Print and shaded views of the part. All mm, measured from the part's lowest x, y and z. Give positions to 0.01 mm unless a question says otherwise; leave off trailing zeros. Loops run counter-clockwise (first coordinate to the right, second up) from the corner with the lowest first, then second, coordinate; pieces in that order, holes last. Notation, with made-up numbers: M -0.75,72.5 L 34.25,72.5 A23 ccw 34.25,111.5 Z; hole C 55.25,89 d10. An arc over 180 degrees is marked long. Put each result on its own line as item: value. Start each with the question number.
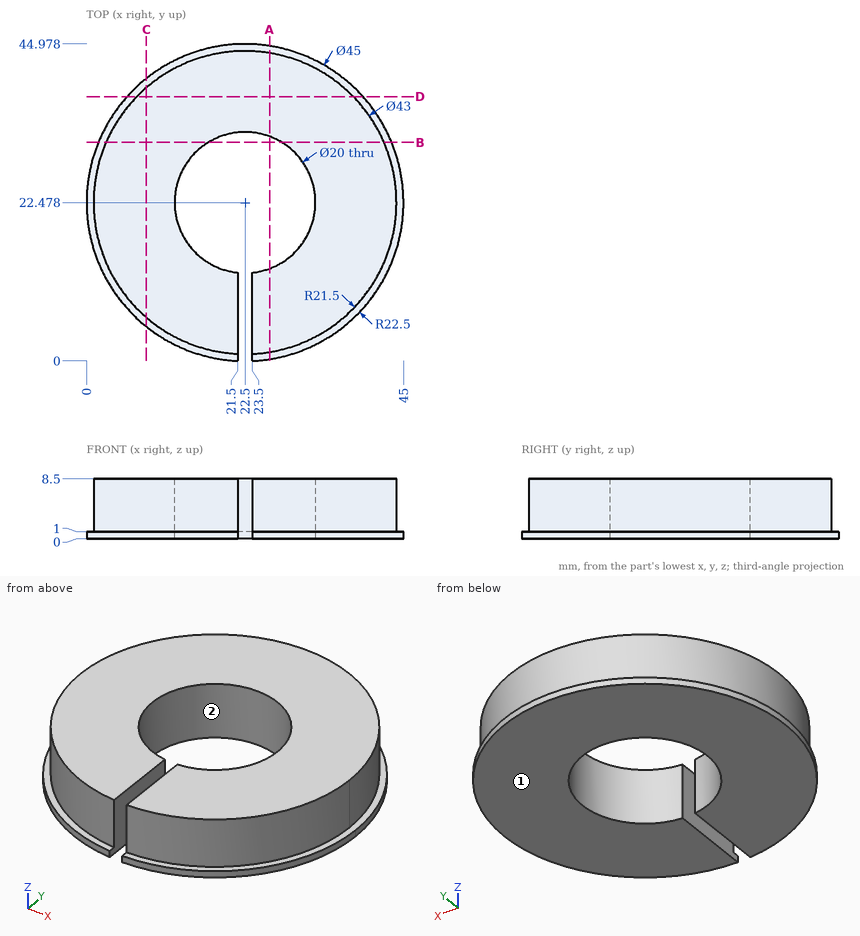
1) Pin check, flat tips, straight feed: pin 1 Ø3 at (y, z) = (9.5, 7.5) entering from +X; pin 2 Ø2.5 at (y, z) = (4.5, 5) entering from +X; pin 3 Ø5 at (x, z) = (32, 5.5) entering from -Y. Stop position of each tip, or through.
2) Wall check: L1, parallel to X at y = 31, z = 2.25; L2, parallel to X at y = 25, z = 3; L3, parallel to Y at x = 29, z = 6.75 (1 decimal). Give the ranges that are in metal, low to high.
3) Band-saw the part on B-B on y = 31. Give the cut face in (x, z), then the cut area to 3 significant figures.
4) Band-saw the part on D-D on y = 37.5. Give the cut face in (x, z), then the cut area to 3 significant figures.
5) Band-saw the part on A-A on x = 26. Give the cut face in (y, z) (1 decimal), then the cut area to 3 significant figures.
6) Band-saw the part on C-C on x = 8.5. Give the cut face in (y, z) (1 decimal).
7) Mould opens along X. For the marked faces 1 and 2 say: +X half, -X half, draft (parallel to the pull), parting line (faces both ways), or undercut.
Evaluation:
1. pin 1: x = 40.68
1. pin 2: x = 36.01
1. pin 3: y = 2.15
2. L1: 2.76 to 17.27, 27.73 to 42.24
2. L2: 1.15 to 12.82, 32.18 to 43.85
2. L3: 2 to 14.9, 30.1 to 43
3. outline: M 1.68,0 L 17.27,0 L 17.27,8.5 L 2.76,8.5 L 2.76,1 L 1.68,1 Z; M 27.73,0 L 43.32,0 L 43.32,1 L 42.24,1 L 42.24,8.5 L 27.73,8.5 Z
3. area: 249 mm2
4. outline: M 5.75,0 L 39.25,0 L 39.25,1 L 37.88,1 L 37.88,8.5 L 7.12,8.5 L 7.12,1 L 5.75,1 Z
4. area: 264 mm2
5. outline: M 0.3,0 L 13.1,0 L 13.1,8.5 L 1.3,8.5 L 1.3,1 L 0.3,1 Z; M 31.8,0 L 44.7,0 L 44.7,1 L 43.7,1 L 43.7,8.5 L 31.8,8.5 Z
5. area: 203 mm2
6. outline: M 4.9,0 L 40.1,0 L 40.1,1 L 38.8,1 L 38.8,8.5 L 6.2,8.5 L 6.2,1 L 4.9,1 Z
7. face 1: draft
7. face 2: undercut
